```python
from build123d import *

# Parameters (mm, degrees)
SKETCH045_R     = 1.475
SKETCH045_R_2   = 4.1
SKETCH045_R_3   = 1.5
PAD013_DEPTH    = 10
SKETCH047_R     = 11.1
POCKET028_DEPTH = 10.001
SKETCH046_R     = 2.6
POCKET029_DEPTH = 2.2
SKETCH048_R     = 2.6
POCKET030_DEPTH = 2.2


with BuildPart() as part:
    # Sketch045 → Pad013 (new body)
    with BuildSketch(Plane.YZ):
        with BuildLine():
            Line((-21, -21), (-21, 21))
            Line((-21, 21), (-11, 21))
            Line((-11, 21), (-11, 30))
            Line((-11, 30), (11, 30))
            Line((11, 30), (11, 21))
            Line((11, 21), (21, 21))
            Line((21, 21), (21, 10))
            Line((21, 10), (0, 10))
            ThreePointArc((0, 10), (-10, 0), (0, -10))
            Line((21, -10), (0, -10))
            Line((21, -21), (21, -10))
            Line((11, -21), (21, -21))
            Line((11, -30), (11, -21))
            Line((-11, -30), (11, -30))
            Line((-11, -21), (-11, -30))
            Line((-21, -21), (-11, -21))
        make_face()
        with Locations((-15.5, 15.5)):
            Circle(SKETCH045_R, mode=Mode.SUBTRACT)
        with Locations((15.5, 15.5)):
            Circle(SKETCH045_R, mode=Mode.SUBTRACT)
        with Locations((-15.5, -15.5)):
            Circle(SKETCH045_R, mode=Mode.SUBTRACT)
        with Locations((15.5, -15.5)):
            Circle(SKETCH045_R, mode=Mode.SUBTRACT)
        with Locations((-15.5, 0)):
            Circle(SKETCH045_R, mode=Mode.SUBTRACT)
        with Locations((0, 17.5)):
            Circle(SKETCH045_R_2, mode=Mode.SUBTRACT)
        with Locations((0, -17.5)):
            Circle(SKETCH045_R_2, mode=Mode.SUBTRACT)
        with Locations((-6.5, 25.14)):
            Circle(SKETCH045_R_3, mode=Mode.SUBTRACT)
        with Locations((6.5, 25.14)):
            Circle(SKETCH045_R_3, mode=Mode.SUBTRACT)
        with Locations((-6.5, -25.14)):
            Circle(SKETCH045_R_3, mode=Mode.SUBTRACT)
        with Locations((6.5, -25.14)):
            Circle(SKETCH045_R_3, mode=Mode.SUBTRACT)
    extrude(amount=PAD013_DEPTH)

    # Sketch047 → Pocket028 (cut, through all)
    with BuildSketch(Plane.YZ):
        Circle(SKETCH047_R)
    extrude(amount=POCKET028_DEPTH, mode=Mode.SUBTRACT)

    # Sketch046 → Pocket029 (cut)
    with BuildSketch(Plane.YZ.offset(10)):
        with Locations((-6.5, 25.14)):
            Circle(SKETCH046_R)
        with Locations((6.5, 25.14)):
            Circle(SKETCH046_R)
        with Locations((-6.5, -25.14)):
            Circle(SKETCH046_R)
        with Locations((6.5, -25.14)):
            Circle(SKETCH046_R)
    extrude(amount=-POCKET029_DEPTH, mode=Mode.SUBTRACT)

    # Sketch048 → Pocket030 (cut)
    with BuildSketch(Plane.YZ):
        with Locations((-15.5, 15.5)):
            Circle(SKETCH048_R)
        with Locations((-15.5, 0)):
            Circle(SKETCH048_R)
        with Locations((-15.5, -15.5)):
            Circle(SKETCH048_R)
        with Locations((15.5, -15.5)):
            Circle(SKETCH048_R)
        with Locations((15.5, 15.5)):
            Circle(SKETCH048_R)
    extrude(amount=POCKET030_DEPTH, mode=Mode.SUBTRACT)


solid = part.part
```
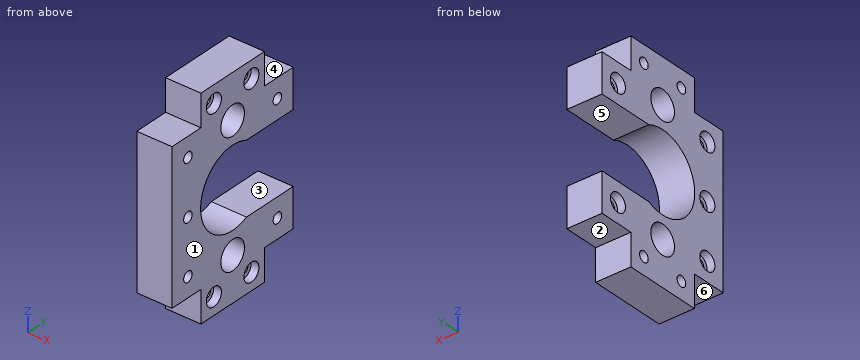
Verification items for the finished model (mm, model axes). Face numbers are marked on the shaded views. A direction names the side the tool comes from. Coordinates: 2 decimals unless noted, no trailing zeros. Order: outer loops, then holes, each group sorted by start corner. A loop starts at its lowest first (then second) coordinate and runs counter-clockwise, first axis right, second up. Notation, with made-up numbers: (44.25, 62.25) -> (90.25, 62.25) arc R15 ccw to (90.25, 90.25) -> close; hole circle Ø4 at (-22.5, 54.5). An arc over 180 degrees is marked (long way). Answer as CSV lines item,"result". Start each with the question number.
1) Cross-section at C-C, the plane x = 6. Give the number of separate pieces and of enclosed holes in the cut face, then the cut area to 3 significant figures.
2) Gauge pin test, flat ends, axial feed: pin 1 Ø3 at (x, y) = (3.5, 16.5) entering from +Z; pin 2 Ø2.5 at (y, z) = (-7.5, -25.5) entering from +X; pin 3 Ø7 at (y, z) = (-6.5, 25.14) entering from -X; pin 4 Ø4.5 at (y, z) = (15.5, 15.5) entering from -X. Record the tip position at first contact, or that the pin passes through.
3) Release check for a two-part mould opening along Z. For the marked faces 1, 2 and 3 record: released by +Z, released by -Z, zero draft, split by the parting line, or undercut.
4) Cross-section at B-B, the plane z = 0. Record the boundary of the cut face in (x, y) (3 decimals).
5) Set-up check for the marked faces 4, 5 and 6: record each of +Z, -Z, +X, -X, +Y, -Y from which the full face is reachable in a straight line by a thin tool's end or side.
6) Cross-section at A-A, the plane y = 6.5. Record the boundary of the cut face in (x, z).
7) Cross-section at D-D, the plane z = -15.5. Record the boundary of the cut face in (x, y) (3 decimals), then the cut area to 3 significant figures.
8) Material ranges on L1, parallel to Y at x = 1.5, z = -25.14; L2, parallel to Z at x = 5.5, y = 0; L3, parallel to Z at x = 4.25, y = 6.5, recorded low to high. Write a range as [from, to].
Conclusion:
1,separate pieces,"1"
1,enclosed holes,"11"
1,area,"1,370 mm²"
2,pin 1,"stops at z = 21"
2,pin 2,"stops at x = 7.8"
2,pin 3,"stops at x = 0"
2,pin 4,"stops at x = 2.2"
3,face 1,"zero draft"
3,face 2,"released by -Z"
3,face 3,"undercut"
4,outline,"(0, -21) -> (10, -21) -> (10, -16.975) -> (2.2, -16.975) -> (2.2, -18.1) -> (0, -18.1) -> close; (0, -12.9) -> (2.2, -12.9) -> (2.2, -14.025) -> (10, -14.025) -> (10, -11.1) -> (0, -11.1) -> close"
5,face 4,"+Z, +X, -X, +Y"
5,face 5,"+X, -X, +Y"
5,face 6,"-Z, +X, -X, -Y"
6,outline,"(0, -30) -> (10, -30) -> (10, -27.74) -> (7.8, -27.74) -> (7.8, -26.64) -> (0, -26.64) -> close; (0, -23.64) -> (7.8, -23.64) -> (7.8, -22.54) -> (10, -22.54) -> (10, -10) -> (0, -10) -> close; (0, 10) -> (10, 10) -> (10, 22.54) -> (7.8, 22.54) -> (7.8, 23.64) -> (0, 23.64) -> close; (0, 26.64) -> (7.8, 26.64) -> (7.8, 27.74) -> (10, 27.74) -> (10, 30) -> (0, 30) -> close"
7,outline,"(0, -21) -> (10, -21) -> (10, -16.975) -> (2.2, -16.975) -> (2.2, -18.1) -> (0, -18.1) -> close; (0, -12.9) -> (2.2, -12.9) -> (2.2, -14.025) -> (10, -14.025) -> (10, -3.579) -> (0, -3.579) -> close; (0, 3.579) -> (10, 3.579) -> (10, 14.025) -> (2.2, 14.025) -> (2.2, 12.9) -> (0, 12.9) -> close; (0, 18.1) -> (2.2, 18.1) -> (2.2, 16.975) -> (10, 16.975) -> (10, 21) -> (0, 21) -> close"
7,area,"280 mm²"
8,L1,"y = [-11, -8], [-5, 5], [8, 11]"
8,L2,"z = [-30, -21.6], [-13.4, -11.1], [11.1, 13.4], [21.6, 30]"
8,L3,"z = [-30, -26.64], [-23.64, -10], [10, 23.64], [26.64, 30]"
